Build history of the part. All positions in model axes, mm. A direction names the side the tool comes from. Round coordinates to 2 decimals unless told otherwise and drop trailing zeros. Write each loop counter-clockwise with the first axis right and the second up, starting at its lowest first coordinate (ties: lowest second). Pieces come first, ordered by that corner, then holes. Notation, with made-up numbers: (67, 85) -> (97, 85) arc R27 ccw to (97, 120) -> close; hole circle Ø9 at (55, -19.75). An arc over 180 degrees is marked (long way). Answer in a Markdown table with one row per item.
```python
from build123d import *

# Parameters (mm, degrees)
BOSS_EXTRUDE1_DEPTH = 12


with BuildPart() as part:
    # Sketch1 → Boss-Extrude1 (new body)
    with BuildSketch(Plane.XY):
        with BuildLine():
            Line((-4.455735931, 20.3), (-3.25, 20.3))
            Line((-3.25, 20.3), (-3.25, 23.3))
            Line((-3.25, 23.3), (-4.455735931, 23.3))
            Line((-4.455735931, 23.3), (-9.5, 23.3))
            ThreePointArc((-9.5, 23.3), (-12.187005769, 22.187005769), (-13.3, 19.5))
            Line((-13.3, 19.5), (-13.3, 14.455735931))
            Line((-13.3, 14.455735931), (-13.3, 5.544264069))
            Line((-13.3, 5.544264069), (-13.3, -5.544264069))
            Line((-13.3, -5.544264069), (-13.3, -14.455735931))
            Line((-13.3, -14.455735931), (-13.3, -19.5))
            ThreePointArc((-13.3, -19.5), (-12.187005769, -22.187005769), (-9.5, -23.3))
            Line((-9.5, -23.3), (-4.455735931, -23.3))
            Line((-4.455735931, -23.3), (4.455735931, -23.3))
            Line((4.455735931, -23.3), (9.5, -23.3))
            ThreePointArc((9.5, -23.3), (12.187005769, -22.187005769), (13.3, -19.5))
            Line((13.3, -19.5), (13.3, -14.455735931))
            Line((13.3, -14.455735931), (13.3, -5.544264069))
            Line((13.3, -5.544264069), (13.3, 5.544264069))
            Line((13.3, 5.544264069), (13.3, 14.455735931))
            Line((13.3, 14.455735931), (13.3, 19.5))
            ThreePointArc((13.3, 19.5), (12.187005769, 22.187005769), (9.5, 23.3))
            Line((9.5, 23.3), (4.455735931, 23.3))
            Line((4.455735931, 23.3), (3.25, 23.3))
            Line((3.25, 23.3), (3.25, 20.3))
            Line((3.25, 20.3), (4.455735931, 20.3))
            Line((4.455735931, 20.3), (9.5, 20.3))
            ThreePointArc((9.5, 20.3), (10.065685425, 20.065685425), (10.3, 19.5))
            Line((10.3, 19.5), (10.3, 14.455735931))
            Line((10.3, 14.455735931), (10.3, 5.544264069))
            Line((10.3, 5.544264069), (10.3, -5.544264069))
            Line((10.3, -5.544264069), (10.3, -14.455735931))
            Line((10.3, -14.455735931), (10.3, -19.5))
            ThreePointArc((10.3, -19.5), (10.065685425, -20.065685425), (9.5, -20.3))
            Line((9.5, -20.3), (4.455735931, -20.3))
            Line((4.455735931, -20.3), (-4.455735931, -20.3))
            Line((-4.455735931, -20.3), (-9.5, -20.3))
            ThreePointArc((-9.5, -20.3), (-10.065685425, -20.065685425), (-10.3, -19.5))
            Line((-10.3, -19.5), (-10.3, -14.455735931))
            Line((-10.3, -14.455735931), (-10.3, -5.544264069))
            Line((-10.3, -5.544264069), (-10.3, 5.544264069))
            Line((-10.3, 5.544264069), (-10.3, 14.455735931))
            Line((-10.3, 14.455735931), (-10.3, 19.5))
            ThreePointArc((-10.3, 19.5), (-10.065685425, 20.065685425), (-9.5, 20.3))
            Line((-9.5, 20.3), (-4.455735931, 20.3))
        make_face()
    extrude(amount=-BOSS_EXTRUDE1_DEPTH)


solid = part.part
```
Q1. Drop flat-ended pins along their axis: P1, Ø2.5, axis at y = 21, z = -5.5, coming from the +X side; P2, Ø1, axis at x = -1.5, z = -4, coming from the +Y side; P3, Ø0.9, axis at y = 22.5, z = -5.5, coming from the -X side. Give the stop position or say it passes through.
A:
| item | result |
|---|---|
| P1 | x = 13.29 |
| P2 | y = -20.3 |
| P3 | x = -12.32 |
Q2. Which spindle directions (+Z, -Z, +X, -X, +Y, -Y) get a long thin tool onto all of the face, cutting with end or side? Do faces 1 (the flat face through (-6, 23.3, -6)), 2 (the flat face through (-3.25, 22, -6)), 3 (the flat face through (6, 20.3, -6)). Say none if no direction does.
A:
| item | result |
|---|---|
| face 1 | +Z, -Z, +X, -X, +Y |
| face 2 | +Z, -Z, +Y |
| face 3 | +Z, -Z |
Q3. Saw through at B-B on y = 6. Write the cut outline in (x, z).
A:
| item | result |
|---|---|
| outline | (-13.3, -12) -> (-10.3, -12) -> (-10.3, 0) -> (-13.3, 0) -> close; (10.3, -12) -> (13.3, -12) -> (13.3, 0) -> (10.3, 0) -> close |
Q4. Saw through at C-C on z = -6.5. Write the cut outline in (x, y).
A:
| item | result |
|---|---|
| outline | (-13.3, -19.5) arc R3.8 ccw to (-9.5, -23.3) -> (9.5, -23.3) arc R3.8 ccw to (13.3, -19.5) -> (13.3, 19.5) arc R3.8 ccw to (9.5, 23.3) -> (3.25, 23.3) -> (3.25, 20.3) -> (9.5, 20.3) arc R0.8 cw to (10.3, 19.5) -> (10.3, -19.5) arc R0.8 cw to (9.5, -20.3) -> (-9.5, -20.3) arc R0.8 cw to (-10.3, -19.5) -> (-10.3, 19.5) arc R0.8 cw to (-9.5, 20.3) -> (-3.25, 20.3) -> (-3.25, 23.3) -> (-9.5, 23.3) arc R3.8 ccw to (-13.3, 19.5) -> close |
Q5. Two-plate mould, pull along X, no slides. Class faces 4 (the flat face through (-10.3, 0, -6)), 5 (the flat face through (0, -23.3, -6)), 6 (the cylindrical face through (12.157, -22.216, -5.916)): released by +X, released by -X, zero draft, split by the parting line, or undercut.
A:
| item | result |
|---|---|
| face 4 | undercut |
| face 5 | zero draft |
| face 6 | released by +X |
Q6. Saw through at D-D on x = -2.75. Write the cut outline in (y, z), plus the area to 3 significant figures.
A:
| item | result |
|---|---|
| outline | (-23.3, -12) -> (-20.3, -12) -> (-20.3, 0) -> (-23.3, 0) -> close |
| area | 36.0 mm² |
Q7. Saw through at A-A on x = 7.5. Write the cut outline in (y, z).
A:
| item | result |
|---|---|
| outline | (-23.3, -12) -> (-20.3, -12) -> (-20.3, 0) -> (-23.3, 0) -> close; (20.3, -12) -> (23.3, -12) -> (23.3, 0) -> (20.3, 0) -> close |
Q8. Wall check: line 1 (X direction, y = -14.5, z = -10.25); line 2 (Y direction, x = 9.25, z = -3.5); line 3 (X direction, y = -20, z = -5.5). Give the ranges that are in metal, low to high. Write a range as [from, to].
A:
| item | result |
|---|---|
| line 1 | [-13.3, -10.3], [10.3, 13.3] |
| line 2 | [-23.3, -20.3], [20.3, 23.3] |
| line 3 | [-13.27, -10.12], [10.12, 13.27] |
